from build123d import *

# Parameters (mm, degrees)
SKETCH_2_R      = 1.25
EXTRUDE_1_DEPTH = 1.7


with BuildPart() as part:
    # Эскиз2 → Бобышка-Вытянуть1 (new body)
    with BuildSketch(Plane.XY):
        with BuildLine():
            Line((0, 16.5), (0, 20.4))
            ThreePointArc((0, 20.4), (-18.247161486, 7.202535297), (-11.42657443, -14.259327835))
            ThreePointArc((-11.42657443, -14.259327835), (-10.414964854, -15.583182123), (-10.265681334, -17.242597243))
            ThreePointArc((-10.265681334, -17.242597243), (-7.750266266, -20.566241003), (-4.717815883, -17.706491802))
            Line((-4.717815883, -17.706491802), (-4.730782246, -17.182866897))
            ThreePointArc((-4.730782246, -17.182866897), (-5.092718531, -16.084006582), (-6.002583463, -15.369417418))
            ThreePointArc((-6.002583463, -15.369417418), (-16.21489111, 3.054063899), (0, 16.5))
        make_face()
        with Locations((-7.516953538, -17.77597844)):
            Circle(SKETCH_2_R, mode=Mode.SUBTRACT)
    extrude(amount=EXTRUDE_1_DEPTH)

    # Зеркальное отражение1: part across plane


with BuildPart() as part_1:
    add(part.part)
    add(part.part.mirror(Plane(origin=(0, 16.5, 1.7), x_dir=(0, 0, 1), z_dir=(-1, 0, 0))))


solid = part_1.part
Could you check a few things on this model? Use its own coordinates, in mm. A direction names the side the tool comes from. Coordinates: 2 decimals unless noted, no trailing zeros. Loops run counter-clockwise (first coordinate to the right, second up) from the corner with the lowest first, then second, coordinate; pieces in that order, holes last.
1. Imagine slicing it at A-A (x = 13.5). Please give me the cut outline in (y, z), and give its area (3 significant figures).
2. Imagine slicing it at D-D (x = -8). Please give me the cut outline in (y, z), and give its area (3 significant figures).
3. I need wall thicknesses on L1, parallel to Y at x = -7.5, z = 1.6; L2, parallel to Y at x = 5, z = 1.2; L3, parallel to Y at x = 13, z = 1.55. Which ranges of each line are inside material? Lowest first, please.
4. We'd pull the mould along Y, two halves only. Please class faces 1 (the face through (-1, 17, 1.7)), 2 (the face through (-10.424, -15.561, 0.838)): released by +Y, released by -Y, zero draft, split by the parting line, or undercut.
5. Imagine slicing it at B-B (y = 1.5). Please give me the cut outline in (x, z), and give its area (3 significant figures).
6. For faces 3 (the face through (-1, 17, 0)), 4 (the face through (-5.08, -16.1, 0.84)), which set-ups out of +Z, -Z, +X, -X, +Y, -Y let a thin tool reach every point of the face, with its end or its side?
7. Imagine slicing it at C-C (z = 0.6). Please give me the cut outline in (x, y), and give its area (3 significant figures).
8. For P1, Ø1, axis at y = -1.5, z = 1, coming from the +X side, with a flat end and sliding along its axis, tell me the tip position at first contact or that it passes through.
Computed values:
1. outline: (-12.48, 0) - (-9.49, 0) - (-9.49, 1.7) - (-12.48, 1.7) - close; (9.49, 0) - (14.86, 0) - (14.86, 1.7) - (9.49, 1.7) - close
1. area: 14.2 mm2
2. outline: (-20.53, 0) - (-18.93, 0) - (-18.93, 1.7) - (-20.53, 1.7) - close; (-16.62, 0) - (-14.43, 0) - (-14.43, 1.7) - (-16.62, 1.7) - close; (14.43, 0) - (18.66, 0) - (18.66, 1.7) - (14.43, 1.7) - close
2. area: 13.6 mm2
3. L1: y = -20.58 to -19.03, -16.53 to -14.7, 14.7 to 18.88
3. L2: y = -19 to -16.23, 15.72 to 19.74
3. L3: y = -12.96 to -10.16, 10.16 to 15.33
4. face 1: zero draft
4. face 2: undercut
5. outline: (-19.21, 0) - (-16.43, 0) - (-16.43, 1.7) - (-19.21, 1.7) - close; (16.43, 0) - (19.21, 0) - (19.21, 1.7) - (16.43, 1.7) - close
5. area: 9.45 mm2
6. face 3: -Z, +X, -X, +Y, -Y
6. face 4: +Z, -Z
7. outline: (-11.43, -14.26) arc R3 cw to (-10.27, -17.24) arc R2.8 ccw (long way) to (-4.72, -17.71) - (-4.73, -17.18) arc R2 ccw to (-6, -15.37) arc R16.5 cw (long way) to (6, -15.37) arc R2 ccw to (4.73, -17.18) - (4.72, -17.71) arc R2.8 ccw (long way) to (10.27, -17.24) arc R3 cw to (11.43, -14.26) arc R19.21 ccw (long way) to start; hole circle Ø2.5 at (-7.52, -17.78); hole circle Ø2.5 at (7.52, -17.78)
7. area: 319 mm2
8. P1: stops at x = 19.09
